Part model, mm, in its own coordinate system. Round coordinates to 2 decimals unless told otherwise and drop trailing zeros. Loops run counter-clockwise (first coordinate to the right, second up) from the corner with the lowest first, then second, coordinate; pieces in that order, holes last.
(1) Flat gauge pins, fed straight in: pin 1 (1.5 mm diameter, centred on y = 22, z = 1.5, fed in from -X); pin 2 (1.5 mm diameter, centred on x = -427, z = 3, fed in from +Y). Where does each tip first touch, or does it go through?
(2) Mould opens along X. For faces 1 (the face through (-222, 82, 0)), 2 (the face through (-220.23, 101.5, 2.46)) say: +X half, -X half, draft (parallel to the pull), parting line (faces both ways), or undercut.
(3) Cut at B-B on x = -225. List the corners of the cut face in (y, z), then the cut area to 3 significant figures.
(4) Probe probe 1 along X at (y, z) = (25.5, 2.4); probe 2 along Y at (x, z) = (-225, 3.95); probe 3 along X at (y, z) = (93, 1.5). List the from-to ranges inside material, lowest first.
(5) Cut at A-A on y = 100. List the corners of the cut face in (x, z).
(6) Cut at C-C on z = 1.05. Count the separate pieces of the cut face and the enclosed holes in it, then the cut area to 3 significant figures.
from build123d import *

# Parameters (mm, degrees)
SKETCH1_R           = 5
SKETCH1_W           = 10
SKETCH1_H           = 5
SKETCH1_W_2         = 4.999728605
SKETCH1_H_2         = 10
SKETCH1_W_3         = 5
SKETCH1_H_3         = 20
SKETCH1_W_4         = 25
BOSS_EXTRUDE1_DEPTH = 5


with BuildPart() as part:
    # Sketch1 → Boss-Extrude1 (new body)
    with BuildSketch(Plane.XY):
        Polygon((-5, 5), (-17.5, 5), (-17.5, 10), (-27.5, 10), (-27.5, 5), (-422.5, 5), (-422.5, 10), (-432.5, 10), (-432.5, 5), (-445, 5), (-445, 17.5), (-440, 17.5), (-440, 27.5), (-445, 27.5), (-445, 177.5), (-440, 177.5), (-440, 187.5), (-445, 187.5), (-445, 200), (-432.5, 200), (-432.5, 195), (-422.5, 195), (-422.5, 200), (-27.5, 200), (-27.5, 195), (-17.5, 195), (-17.5, 200), (-5, 200), (-5, 187.5), (-10, 187.5), (-10, 177.5), (-5, 177.5), (-5, 27.5), (-10, 27.5), (-10, 17.5), (-5, 17.5), align=None)
        with Locations((-225, 170)):
            Circle(SKETCH1_R, mode=Mode.SUBTRACT)
        with Locations((-225, 100)):
            Circle(SKETCH1_R, mode=Mode.SUBTRACT)
        with Locations((-22.5, 37.5)):
            Rectangle(SKETCH1_W, SKETCH1_H, mode=Mode.SUBTRACT)
        with Locations((-37.500135697, 22.5)):
            Rectangle(SKETCH1_W_2, SKETCH1_H_2, mode=Mode.SUBTRACT)
        with Locations((-412.499864302, 22.5)):
            Rectangle(SKETCH1_W_2, SKETCH1_H_2, mode=Mode.SUBTRACT)
        with Locations((-427.5, 37.5)):
            Rectangle(SKETCH1_W, SKETCH1_H, mode=Mode.SUBTRACT)
        with Locations((-427.5, 167.5)):
            Rectangle(SKETCH1_W, SKETCH1_H, mode=Mode.SUBTRACT)
        with Locations((-412.499864302, 182.5)):
            Rectangle(SKETCH1_W_2, SKETCH1_H_2, mode=Mode.SUBTRACT)
        with Locations((-37.500135697, 182.5)):
            Rectangle(SKETCH1_W_2, SKETCH1_H_2, mode=Mode.SUBTRACT)
        with Locations((-22.5, 167.5)):
            Rectangle(SKETCH1_W, SKETCH1_H, mode=Mode.SUBTRACT)
        with Locations((-427.5, 67.5)):
            Rectangle(SKETCH1_W_3, SKETCH1_H_3, mode=Mode.SUBTRACT)
        with Locations((-427.5, 102.5)):
            Rectangle(SKETCH1_W_3, SKETCH1_H_3, mode=Mode.SUBTRACT)
        with Locations((-427.5, 137.5)):
            Rectangle(SKETCH1_W_3, SKETCH1_H_3, mode=Mode.SUBTRACT)
        with Locations((-22.5, 137.5)):
            Rectangle(SKETCH1_W_3, SKETCH1_H_3, mode=Mode.SUBTRACT)
        with Locations((-22.5, 102.5)):
            Rectangle(SKETCH1_W_3, SKETCH1_H_3, mode=Mode.SUBTRACT)
        with Locations((-22.5, 67.5)):
            Rectangle(SKETCH1_W_3, SKETCH1_H_3, mode=Mode.SUBTRACT)
        with Locations((-365, 22.5)):
            Rectangle(SKETCH1_W_4, SKETCH1_H, mode=Mode.SUBTRACT)
        with Locations((-295, 22.5)):
            Rectangle(SKETCH1_W_4, SKETCH1_H, mode=Mode.SUBTRACT)
        with Locations((-225, 22.5)):
            Rectangle(SKETCH1_W_4, SKETCH1_H, mode=Mode.SUBTRACT)
        with Locations((-155, 22.5)):
            Rectangle(SKETCH1_W_4, SKETCH1_H, mode=Mode.SUBTRACT)
        with Locations((-85, 22.5)):
            Rectangle(SKETCH1_W_4, SKETCH1_H, mode=Mode.SUBTRACT)
    extrude(amount=BOSS_EXTRUDE1_DEPTH)


solid = part.part
Final values:
1. pin 1: stops at x = -440
1. pin 2: stops at y = 195
2. face 1: draft
2. face 2: undercut
3. outline: (5, 0) - (20, 0) - (20, 5) - (5, 5) - close; (25, 0) - (95, 0) - (95, 5) - (25, 5) - close; (105, 0) - (165, 0) - (165, 5) - (105, 5) - close; (175, 0) - (200, 0) - (200, 5) - (175, 5) - close
3. area: 850 mm2
4. probe 1: x = -440 to -415, -410 to -40, -35 to -10
4. probe 2: y = 5 to 20, 25 to 95, 105 to 165, 175 to 200
4. probe 3: x = -445 to -430, -425 to -25, -20 to -5
5. outline: (-445, 0) - (-430, 0) - (-430, 5) - (-445, 5) - close; (-425, 0) - (-230, 0) - (-230, 5) - (-425, 5) - close; (-220, 0) - (-25, 0) - (-25, 5) - (-220, 5) - close; (-20, 0) - (-5, 0) - (-5, 5) - (-20, 5) - close
6. separate pieces: 1
6. enclosed holes: 21
6. area: 83,600 mm2
